Could you check a few things on this drawing? It's one solid part, dimensions in mm from its lowest x, y, z. Coordinates: 2 decimals unless noted, no trailing zeros. Write each loop counter-clockwise with the first axis right and the second up, starting at its lowest first coordinate (ties: lowest second). Pieces come first, ordered by that corner, then holes. Notation, with made-up numbers: (52, 4.25) - (107, 4.25) arc R17 ccw to (107, 21.25) - close; hole circle Ø10 at (-12.75, 86.25). An arc over 180 degrees is marked (long way). Use one line per item in the form item = value. Start each with the question number.
(1) If we section it at A-A on z = 13: Please give me the cut outline in (x, y).
(2) If we section it at D-D on z = 19.5: Please give me the cut outline in (x, y), then the cut area to 3 significant figures.
(3) If I drill on probe 1 along X at (y, z) = (3.1, 13); probe 2 along Z at (x, y) = (29, 1.25); probe 3 along Z at (x, y) = (15.5, 1.25), over which ranges is the centre line in solid material (lowest first)? Write a range as from..to.
(4) If we section it at C-C on y = 0.8: Please give me the cut outline in (x, z).
(5) If we section it at B-B on x = 29.1: Please give me the cut outline in (y, z).
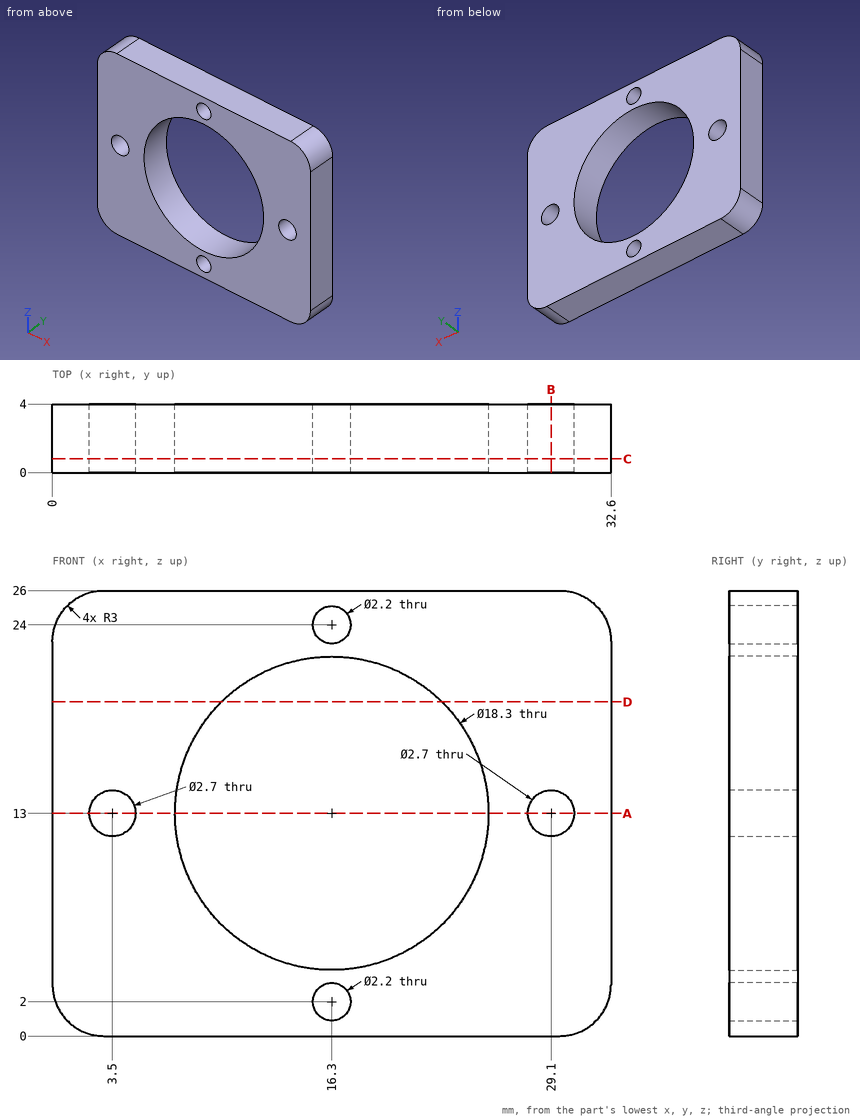
Reported:
q1.outline = (0, 0) - (2.15, 0) - (2.15, 4) - (0, 4) - close; (4.85, 0) - (7.15, 0) - (7.15, 4) - (4.85, 4) - close; (25.45, 0) - (27.75, 0) - (27.75, 4) - (25.45, 4) - close; (30.45, 0) - (32.6, 0) - (32.6, 4) - (30.45, 4) - close
q2.outline = (0, 0) - (9.86, 0) - (9.86, 4) - (0, 4) - close; (22.74, 0) - (32.6, 0) - (32.6, 4) - (22.74, 4) - close
q2.area = 78.9 mm2
q3.probe_1 = 0..2.15, 4.85..7.15, 25.45..27.75, 30.45..32.6
q3.probe_2 = 0..11.65, 14.35..26
q3.probe_3 = 0..1.25, 2.75..3.89, 22.11..23.25, 24.75..26
q4.outline = (0, 3) arc R3 ccw to (3, 0) - (29.6, 0) arc R3 ccw to (32.6, 3) - (32.6, 23) arc R3 ccw to (29.6, 26) - (3, 26) arc R3 ccw to (0, 23) - close; hole circle Ø2.7 at (3.5, 13); hole circle Ø18.3 at (16.3, 13); hole circle Ø2.2 at (16.3, 2); hole circle Ø2.2 at (16.3, 24); hole circle Ø2.7 at (29.1, 13)
q5.outline = (0, 0) - (4, 0) - (4, 11.65) - (0, 11.65) - close; (0, 14.35) - (4, 14.35) - (4, 26) - (0, 26) - close
